```python
from build123d import *

# Parameters (mm, degrees)
F0_W     = 200
F0_H     = 200
F0_W_2   = 162.2
F0_H_2   = 162.2
F1_DEPTH = 200
F2_W     = 200
F2_H     = 200
F3_DEPTH = 200
F4_W     = 200
F4_H     = 200
F5_DEPTH = 650


with BuildPart() as f1:
    # F0 (on Top) → F1 (new body)
    with BuildSketch(Plane.XY):
        Rectangle(F0_W, F0_H)
        Rectangle(F0_W_2, F0_H_2, mode=Mode.SUBTRACT)
    extrude(amount=F1_DEPTH)

    # F2 (on face) → F3 (join)
    with BuildSketch(Plane.XY.offset(200)):
        Rectangle(F2_W, F2_H)
    extrude(amount=F3_DEPTH)

    # F4 (on face) → F5 (join)
    with BuildSketch(Plane.YZ.offset(100)):
        with Locations((0, 300)):
            Rectangle(F4_W, F4_H)
    extrude(amount=F5_DEPTH)


solid = f1.part
```
Verification items for the finished model (mm, model axes). A direction names the side the tool comes from. Coordinates: 2 decimals unless noted, no trailing zeros. Order: outer loops, then holes, each group sorted by start corner. A loop starts at its lowest first (then second) coordinate and runs counter-clockwise, first axis right, second up. Notation, with made-up numbers: (-19.5, 6) - (2.5, 6) arc R31 cw to (2.5, 38) - close; hole circle Ø1 at (58, -16). An arc over 180 degrees is marked (long way). Return JSON: item names as keys, results as strings.
(1) Section check C-C, the plane x = 22. Record the cut outline in (y, z).
Filled sheet:
{"outline": "(-100, 0) - (-81.1, 0) - (-81.1, 200) - (81.1, 200) - (81.1, 0) - (100, 0) - (100, 400) - (-100, 400) - close"}
(2) Section check A-A, the plane y = 10. Record the cut outline in (x, z).
Filled sheet:
{"outline": "(-100, 0) - (-81.1, 0) - (-81.1, 200) - (81.1, 200) - (81.1, 0) - (100, 0) - (100, 200) - (750, 200) - (750, 400) - (-100, 400) - close"}
(3) Go/stop test with flat-tipped pins: pin 1 (3 mm diameter, centred on y = 79, z = 71, fed in from +X); pin 2 (5 mm diameter, centred on x = 646.5, y = -75, fed in from -Z). Record where each tip stops, or that it passes through.
Filled sheet:
{"pin 1": "stops at x = 100", "pin 2": "stops at z = 200"}
(4) Access from +Z, -Z, +X, -X, +Y, -Y to the whole of each face (thin tool, end or side, straight path). Record for faces 1 (the flat face through (-90, 1, 0)), 2 (the flat face through (420, -1, 200)), 3 (the flat face through (81.1, -1, 99)).
Filled sheet:
{"face 1": "-Z, +X, -X, +Y, -Y", "face 2": "-Z, +X, +Y, -Y", "face 3": "-Z"}
(5) Mould release check, pull along Y, two halves, no side actions. Record for faces 4 (the flat face through (750, -1, 301)), 5 (the flat face through (225, -100, 286)), 6 (the flat face through (-1, -81.1, 99)): pulls with the +Y half, pulls with the -Y half, needs draft (parallel to the pull), parting line crosses it, or undercut.
Filled sheet:
{"face 4": "needs draft", "face 5": "pulls with the -Y half", "face 6": "undercut"}
(6) Section check D-D, the plane x = 266.5. Record the cut outline in (y, z), and give its area (3 significant figures).
Filled sheet:
{"outline": "(-100, 200) - (100, 200) - (100, 400) - (-100, 400) - close", "area": "40,000 mm^2"}
(7) Section check B-B, the plane z = 59. Record the cut outline in (x, y), and give its area (3 significant figures).
Filled sheet:
{"outline": "(-100, -100) - (100, -100) - (100, 100) - (-100, 100) - close; hole (-81.1, -81.1) - (81.1, -81.1) - (81.1, 81.1) - (-81.1, 81.1) - close", "area": "13,700 mm^2"}
(8) Thickness scan on line 1 along X through (y, z) = (-15, 173.5); line 2 along Z through (x, y) = (448.5, 46); line 3 along X through (y, z) = (-83.5, 77). Record the ranges inside material, lowest first.
Filled sheet:
{"line 1": "x = -100 to -81.1, 81.1 to 100", "line 2": "z = 200 to 400", "line 3": "x = -100 to 100"}
